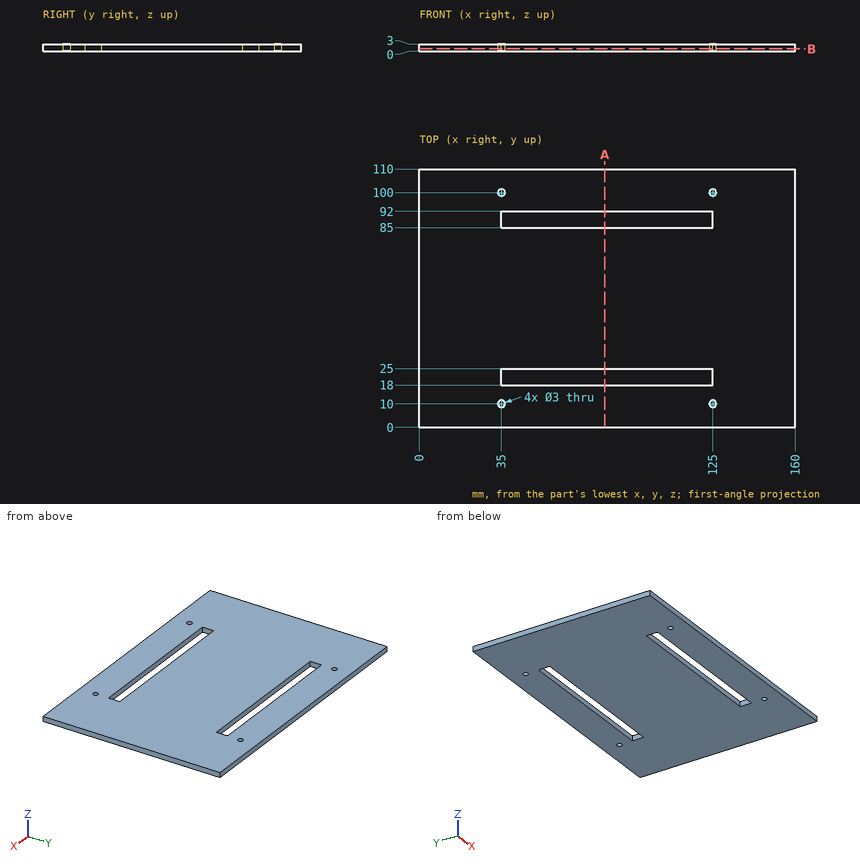
Job drawing, mm, ordinate dimensions from the low corner. One solid piece. Coordinates: 2 decimals unless noted, no trailing zeros. Order: outer loops, then holes, each group sorted by start corner. A loop starts at its lowest first (then second) coordinate and runs counter-clockwise, first axis right, second up. Notation, with made-up numbers: M 33.5,-18 L 62.5,-18 A31 ccw 62.5,17 Z; hole C 76.25,-7.75 d1. An arc over 180 degrees is marked long. Answer as CSV lines item,"result".
(1) Band-saw the part on A-A, the plane x = 79. List the corners of the cut face in (y, z), then the cut area to 3 significant figures.
Geometry says:
outline,"M 0,0 L 18,0 L 18,3 L 0,3 Z; M 25,0 L 85,0 L 85,3 L 25,3 Z; M 92,0 L 110,0 L 110,3 L 92,3 Z"
area,"288 mm2"
(2) Wall check: line 1 along X through (y, z) = (100, 1.8); line 2 along Y through (x, z) = (99.5, 0.3); line 3 along X through (y, z) = (90, 0.6). Give the ranges that are in metal, low to high.
Geometry says:
line 1,"x = 0 to 33.5, 36.5 to 123.5, 126.5 to 160"
line 2,"y = 0 to 18, 25 to 85, 92 to 110"
line 3,"x = 0 to 35, 125 to 160"
(3) Flat gauge pin, fed straight in: pin 1 (6 mm diameter, centred on x = 76.5, y = 22.5, fed in from +Z). Where does the tip first touch, or does it go through?
Geometry says:
pin 1,"stops at z = 3"
(4) Band-saw the part on B-B, the plane z = 0.9. List the corners of the cut face in (x, y).
Geometry says:
outline,"M 0,0 L 160,0 L 160,110 L 0,110 Z; hole C 35,10 d3; hole C 35,100 d3; hole M 35,18 L 125,18 L 125,25 L 35,25 Z; hole M 35,85 L 125,85 L 125,92 L 35,92 Z; hole C 125,10 d3; hole C 125,100 d3"
